Here's the drawing with two shaded views (mm, measured from the low corner). I have some questions. A direction names the side the tool comes from. Coordinates: 2 decimals unless noted, no trailing zeros. Write each loop counter-clockwise with the first axis right and the second up, starting at its lowest first coordinate (ties: lowest second). Pieces come first, ordered by that corner, then holes.
Item 1: If we section it at A-A (x = 9): Please give me the cut outline in (y, z) (1 decimal).
Item 2: I'm going to push flat-ended pins straight in: pin 1 Ø5 at (y, z) = (10.5, 5) entering from -X; pin 2 Ø4.5 at (x, y) = (5, 7.5) entering from +Z; pin 3 Ø6 at (x, z) = (10.5, 1) entering from -Y. Where does each tip first touch, or does it pass through?
Item 3: For the marked faces 4, 5, 6 and 7, which set-ups out of +Z, -Z, +X, -X, +Y, -Y let a thin tool reach every point of the face, with its end or its side?
Item 4: We'd pull the mould along Y, two halves only. Please class the marked faces 1, 2 and 3: +Y half, -Y half, draft (parallel to the pull), parting line (faces both ways), or undercut.
Item 5: If we section it at C-C (z = 1.25): Please give me the cut outline in (x, y) (1 decimal).
Item 6: If we section it at B-B (y = 8.5): Please give me the cut outline in (x, z).
Item 7: If I drill on line 1 (Z direction, x = 4, y = 6.5); line 2 (Z direction, x = 3.25, y = 12); line 3 (X direction, y = 7.5, z = 10.5), over which ranges is the centre line in solid material (lowest first)?
Item 8: If we section it at D-D (y = 3.75): Please give me the cut outline in (x, z).
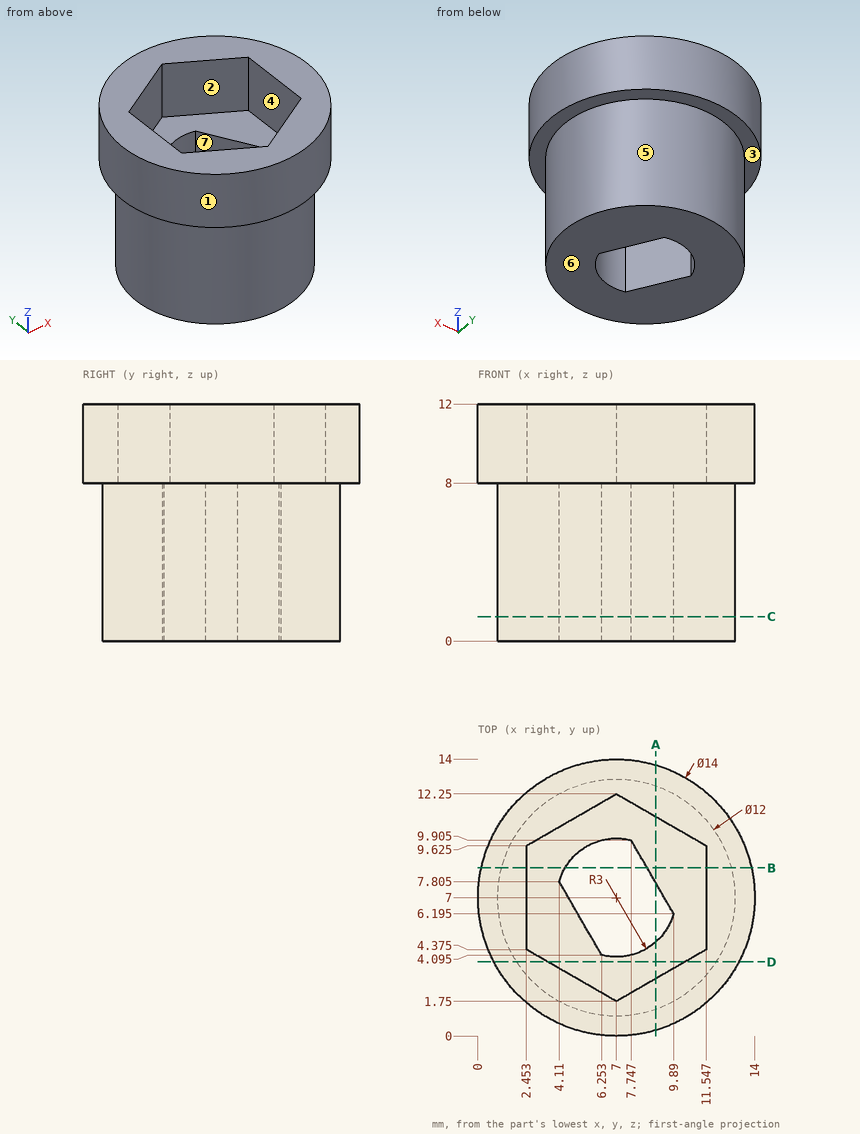
Answer list:
1. outline: (0.3, 8) - (1.3, 8) - (1.3, 0) - (4.8, 0) - (4.8, 8) - (2.9, 8) - (2.9, 12) - (0.3, 12) - close; (7.7, 0) - (12.7, 0) - (12.7, 8) - (13.7, 8) - (13.7, 12) - (11.1, 12) - (11.1, 8) - (7.7, 8) - close
2. pin 1: stops at x = 1.08
2. pin 2: stops at z = 8
2. pin 3: stops at y = 1.02
3. face 4: +Z
3. face 5: -Z
3. face 6: -Z, +X, -X, +Y, -Y
3. face 7: +Z, -Z
4. face 1: parting line
4. face 2: undercut
4. face 3: draft
5. outline: circle Ø12 at (7, 7); hole (4.1, 7.8) - (6.3, 4.1) arc R3 ccw to (9.9, 6.2) - (7.7, 9.9) arc R3 ccw to start
6. outline: (0.16, 8) - (1.19, 8) - (1.19, 0) - (4.4, 0) - (4.4, 8) - (2.45, 8) - (2.45, 12) - (0.16, 12) - close; (8.56, 0) - (12.81, 0) - (12.81, 8) - (13.84, 8) - (13.84, 12) - (11.55, 12) - (11.55, 8) - (8.56, 8) - close
7. line 1: z = 0 to 8
7. line 2: z = 8 to 12
7. line 3: x = 0.02 to 2.45, 11.55 to 13.98
8. outline: (0.8, 8) - (1.96, 8) - (1.96, 0) - (12.04, 0) - (12.04, 8) - (13.2, 8) - (13.2, 12) - (10.46, 12) - (10.46, 8) - (3.54, 8) - (3.54, 12) - (0.8, 12) - close
